Source: CAD feature listing. Evaluate the final solid. Frame: model axes, mm. A direction names the side the tool comes from. Give positions to 0.01 mm unless a question says otherwise; leave off trailing zeros. Write each loop counter-clockwise with the first axis right and the second up, starting at its lowest first coordinate (ties: lowest second). Pieces come first, ordered by that corner, then holes. Notation, with made-up numbers: M 46.25,84.5 L 70.25,84.5 A9 cw 70.25,92.5 Z; hole C 13,32.5 d11. An arc over 180 degrees is marked long. Return JSON: item names as keys, results as strings.
```python
from build123d import *

# Parameters (mm, degrees)
SKETCH1_W           = 38.1
SKETCH1_H           = 43.942
EXTRUDE1_DEPTH      = 45.847
EXTRUDE1_DEPTH_BACK = 25.4
CUT_EXTRUDE1_REACH  = 47.847
SKETCH2_W           = 38.1
SKETCH2_H           = 43.942
SKETCH2_R           = 13.3604
SKETCH14_R          = 7.9375
CUT_EXTRUDE2_DEPTH  = 2.667
SKETCH10_R          = 6.4389
EXTRUDE2_DEPTH      = 1.651
SKETCH11_R          = 4.8006
EXTRUDE3_DEPTH      = 2.667
CIRPATTERN1_COUNT   = 4
HOLE1_D             = 5.5626
HOLE1_DEPTH         = 25.4


with BuildPart() as part:
    # Sketch1 → Extrude1 (new body, two sides)
    with BuildSketch(Plane(origin=(0, 0, 0), x_dir=(0, 0, -1), z_dir=(1, 0, 0))) as extrude1_sk:
        with Locations((0, -8.4836)):
            Rectangle(SKETCH1_W, SKETCH1_H)
    extrude(amount=EXTRUDE1_DEPTH)
    extrude(extrude1_sk.sketch, amount=-EXTRUDE1_DEPTH_BACK)

    # Sketch2 → Cut-Extrude1 (cut, up to next)
    with BuildSketch(Plane(origin=(0, 0, 0), x_dir=(0, 0, -1), z_dir=(1, 0, 0)), mode=Mode.PRIVATE) as cut_extrude1_sk1:
        with Locations((0, -8.4836)):
            Rectangle(SKETCH2_W, SKETCH2_H)
        Circle(SKETCH2_R, mode=Mode.SUBTRACT)
    cut_extrude1_tool1 = extrude(cut_extrude1_sk1.sketch, amount=CUT_EXTRUDE1_REACH, mode=Mode.PRIVATE) & part.part
    add(cut_extrude1_tool1.solids().sort_by_distance((0, 13.429241, 0))[0], mode=Mode.SUBTRACT)

    # Sketch3 → Cut-Revolve1 (revolve, cut)
    with BuildSketch(Plane.XY, mode=Mode.PRIVATE) as cut_revolve1_sk:
        Polygon((42.752748967, 13.3604), (45.847, 8.001), (45.847, 13.3604), align=None)
    revolve(cut_revolve1_sk.sketch.rotate(Axis((42.598036416, 0, 0), (1, 0, 0)), 90), axis=Axis((42.598036416, 0, 0), (1, 0, 0)), mode=Mode.SUBTRACT)  # turned: the seam where the file's is

    # S2D0002 → Cut-Revolve2 (revolve, cut)
    with BuildSketch(Plane(origin=(-22.733, -19.8374, 9.525), x_dir=(0, 1, 0), z_dir=(0, 0, 1)), mode=Mode.PRIVATE) as cut_revolve2_sk:
        Polygon((-0.8128, 0), (3.7338, 0), (3.293786662, -2.0701), (2.6416, -2.722286662), (2.6416, -13.97), (-0.8128, -13.97), align=None)
    revolve(cut_revolve2_sk.sketch.rotate(Axis((-8.0645, -20.6502, 9.525), (-1, 0, 0)), 90), axis=Axis((-8.0645, -20.6502, 9.525), (-1, 0, 0)), mode=Mode.SUBTRACT)  # turned: the seam where the file's is

    # Sketch5 → Cut-Revolve3 (revolve, cut)
    with BuildSketch(Plane(origin=(-22.733, -19.8374, -9.525), x_dir=(0, 1, 0), z_dir=(0, 0, 1)), mode=Mode.PRIVATE) as cut_revolve3_sk:
        Polygon((-0.8128, 0), (3.7338, 0), (3.293786662, -2.0701), (2.6416, -2.722286662), (2.6416, -13.97), (-0.8128, -13.97), align=None)
    revolve(cut_revolve3_sk.sketch.rotate(Axis((-8.0645, -20.6502, -9.525), (-1, 0, 0)), 90), axis=Axis((-8.0645, -20.6502, -9.525), (-1, 0, 0)), mode=Mode.SUBTRACT)  # turned: the seam where the file's is

    # Sketch14 → Cut-Extrude2 (cut)
    with BuildSketch(Plane.ZY.offset(25.4)):
        with Locations((-9.525, -20.6502)):
            Circle(SKETCH14_R)
        with Locations((9.525, -20.6502)):
            Circle(SKETCH14_R)
    extrude(amount=-CUT_EXTRUDE2_DEPTH, mode=Mode.SUBTRACT)

    # Sketch6 → Cut-Revolve4 (revolve, cut)
    with BuildSketch(Plane(origin=(-8.7376, -30.2006, 9.525), x_dir=(-1, 0, 0), z_dir=(0, 0, 1)), mode=Mode.PRIVATE) as cut_revolve4_sk:
        Polygon((6.18363, 0), (5.641036865, -2.5527), (4.97713, -3.216606865), (4.97713, -17.272), (0, -17.272), (0, 0), (0, 0.254), (9.52373, 0.254), (9.52373, 0), align=None)
    revolve(cut_revolve4_sk.sketch.rotate(Axis((-8.7376, -12.065, 9.525), (0, -1, 0)), 270), axis=Axis((-8.7376, -12.065, 9.525), (0, -1, 0)), mode=Mode.SUBTRACT)  # turned: the seam where the file's is

    # Sketch7 → Cut-Revolve5 (revolve, cut)
    with BuildSketch(Plane(origin=(-8.7376, -30.2006, -9.525), x_dir=(-1, 0, 0), z_dir=(0, 0, 1)), mode=Mode.PRIVATE) as cut_revolve5_sk:
        Polygon((6.1849, 0), (5.642306865, -2.5527), (4.9784, -3.216606865), (4.9784, -17.272), (0, -17.272), (0, 0), (0, 0.254), (9.52373, 0.254), (9.52373, 0), align=None)
    revolve(cut_revolve5_sk.sketch.rotate(Axis((-8.7376, -12.065, -9.525), (0, -1, 0)), 270), axis=Axis((-8.7376, -12.065, -9.525), (0, -1, 0)), mode=Mode.SUBTRACT)  # turned: the seam where the file's is

    # Sketch8 → Revolve1 (revolve)
    with BuildSketch(Plane.XY, mode=Mode.PRIVATE) as revolve1_sk:
        with BuildLine():
            Line((45.847, 0), (45.847, 5.55625))
            Line((45.847, 5.55625), (65.1256, 5.55625))
            ThreePointArc((65.1256, 5.55625), (65.84402049, 5.25867049), (66.1416, 4.54025))
            Line((66.1416, 4.54025), (66.1416, 0))
            Line((66.1416, 0), (45.847, 0))
        make_face()
    revolve(revolve1_sk.sketch.rotate(Axis((44.83227, 0, 0), (1, 0, 0)), 90), axis=Axis((44.83227, 0, 0), (1, 0, 0)))  # turned: the seam where the file's is

    # S2D0001 → Cut-Revolve6 (revolve, cut)
    with BuildSketch(Plane(origin=(66.1416, -2.8067, 0), x_dir=(0, -1, 0), z_dir=(0, 0, 1)), mode=Mode.PRIVATE) as cut_revolve6_sk:
        Polygon((-0.1016, 0), (-0.1016, -9.652), (-2.8067, -11.277388061), (-2.8067, 0), align=None)
    revolve(cut_revolve6_sk.sketch.rotate(Axis((53.702842726, 0, 0), (1, 0, 0)), 270), axis=Axis((53.702842726, 0, 0), (1, 0, 0)), mode=Mode.SUBTRACT)  # turned: the seam where the file's is

    # Sketch10 → Extrude2 (add)
    with BuildSketch(Plane(origin=(-25.4, -30.2006, 0), x_dir=(0, 0, -1), z_dir=(0, -1, 0))):
        with Locations(Location((-9.525, 16.6624, 0), (0, 0, 180))):  # turned: the seam where the file's is
            Circle(SKETCH10_R)
    extrude(amount=EXTRUDE2_DEPTH)

    # Sketch11 → Extrude3 (add)
    with BuildSketch(Plane.ZY.offset(22.733)):
        with Locations(Location((9.525, -20.6502, 0), (0, 0, 180))):  # turned: the seam where the file's is
            Circle(SKETCH11_R)
    extrude(amount=EXTRUDE3_DEPTH)

    # Sketch12 → Cut-Revolve7 (revolve, cut)
    with BuildSketch(Plane(origin=(62.1792, 3.928862053, -3.928862053), x_dir=(-1, 0, 0), z_dir=(0, -0.707106781, -0.707106781)), mode=Mode.PRIVATE) as cut_revolve7_sk:
        Polygon((0, 0), (1.5875, 0), (0, -1.5875), align=None)
    cut_revolve7 = revolve(cut_revolve7_sk.sketch.rotate(Axis((62.1792, 1.500688387, -1.500688387), (0, 0.707106781, -0.707106781)), 90), axis=Axis((62.1792, 1.500688387, -1.500688387), (0, 0.707106781, -0.707106781)), mode=Mode.SUBTRACT)  # turned: the seam where the file's is

    # CirPattern1: Cut-Revolve7 ×4 about axis
    cirpattern1_axis = Axis((45.848, 0, 0), (-1, 0, 0))
    for i in range(1, CIRPATTERN1_COUNT):
        add(cut_revolve7.rotate(cirpattern1_axis, i * 360 / CIRPATTERN1_COUNT), mode=Mode.SUBTRACT)

    # Hole1
    with Locations(Plane(origin=(0, 0, 0), x_dir=(0, 0, -1), z_dir=(1, 0, 0))):
        with Locations((-15.0876, 9.525), (-15.0876, -9.525), (15.0876, 9.525), (15.0876, -9.525), (0, -26.9748)):
            Hole(HOLE1_D / 2, depth=HOLE1_DEPTH)


solid = part.part
```
1) Contact query for flat-ended pins moving along their axis: pin 1 Ø4.5 at (y, z) = (-21.5, 8.5) entering from +X; pin 2 Ø7.5 at (x, z) = (-15.5, 1) entering from -Y; pin 3 Ø8 at (y, z) = (-0.5, -9) entering from +X. Output: stop coordinate, or through.
Numbers:
{"pin 1": "stops at x = 0", "pin 2": "stops at y = -30.45", "pin 3": "stops at x = 66.02"}
2) Cut plane A-A, the plane x = 25. Return the cut outline in (y, z), then the cut area to 3 significant figures.
Numbers:
{"outline": "C 0,0 d26.72", "area": "561 mm²"}
3) Cut plane B-B, the plane y = 10.5. Give the number of separate pieces and of enclosed holes in the cut face, then the cut area to 3 significant figures.
Numbers:
{"separate pieces": "3", "enclosed holes": "0", "area": "1,430 mm²"}
4) Set-up query: faces 1 (the face through (66.142, 3, 0)), 2 (the face through (-15.3, -30.201, -9.7)), 3 (the face through (-22.733, -24, -6)). Return all of +Z, -Z, +X, -X, +Y, -Y with unobstructed straight access to the full face (end or side cutting, diameter ignored); none if empty.
Numbers:
{"face 1": "+Z, -Z, +X, +Y, -Y", "face 2": "-Y", "face 3": "-X"}
5) Draft query along X for faces 4 (the face through (-12.878, -9.403, -17.866)), 5 (the face through (-9, -12.929, 9)), 6 (the face through (55.12, 0.42, -0.09)), 7 (the face through (-22.733, -21, 15)). Return one class per face: released by +X, released by -X, zero draft, split by the parting line, or undercut.
Numbers:
{"face 4": "zero draft", "face 5": "undercut", "face 6": "released by +X", "face 7": "released by -X"}
6) Line query: line 1 (Y direction, x = 60, z = 0); line 2 (Y direction, x = -18, z = -9.5); line 3 (Y direction, x = -1, z = 13). Output: solid intervals per line, ascending. Write a range as [from, to].
Numbers:
{"line 1": "y = [-5.56, -2.71], [2.71, 5.56]", "line 2": "y = [-30.2, -24.1], [-17.2, 13.49]", "line 3": "y = [-30.2, -11.36], [-7.69, 7.69], [11.36, 13.49]"}
